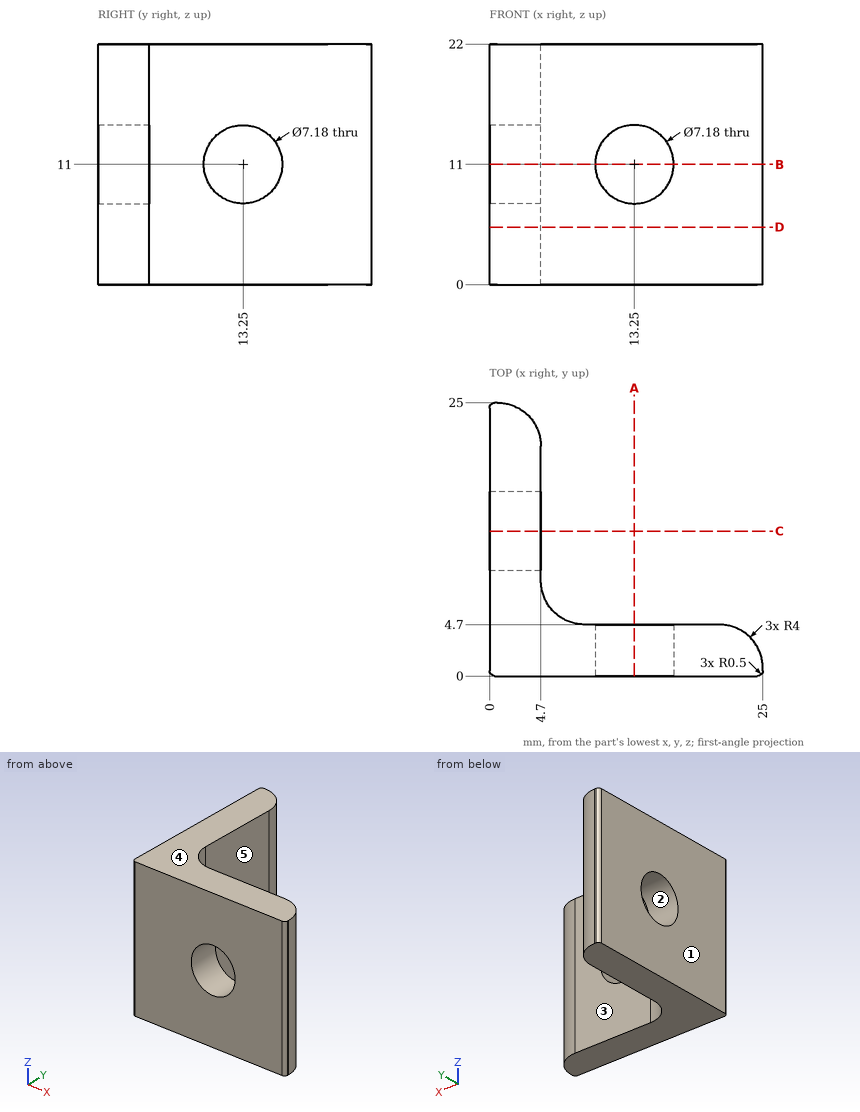
Source: three-view drawing plus pictorial views. Frame: mm from the lowest corner of the part. A direction names the side the tool comes from. Round coordinates to 2 decimals unless told otherwise and drop trailing zeros. Loops run counter-clockwise (first coordinate to the right, second up) from the corner with the lowest first, then second, coordinate; pieces in that order, holes last.
1. Contact query for flat-ended pins moving along their axis: pin 1 (5 mm diameter, centred on y = 16, z = 8, fed in from +X); pin 2 (4 mm diameter, centred on x = 8.5, z = 14.5, fed in from +Y); pin 3 (3.5 mm diameter, centred on x = 17, z = 11, fed in from +Y); pin 4 (5 mm diameter, centred on x = 19, y = 3, fed in from -Z). Output: stop coordinate, or through.
2. Mould query, pull axis Y, two halves, no side actions, for the marked faces 1, 2 and 3. Classes: released by +Y, released by -Y, zero draft, split by the parting line, or undercut.
3. Section query D-D on z = 5.25. Output: boundary loops of the cut face in (x, y), and give its area (3 significant figures).
4. Section query A-A on x = 13.25. Output: boundary loops of the cut face in (y, z).
5. Section query B-B on z = 11. Output: boundary loops of the cut face in (x, y).
6. Ray query, L1, parallel to Z at x = 3.05, y = 13.25; L2, parallel to X at y = 19.75, z = 6.75. Return the intervals inside material, ascending.
7. Access query for the marked faces 4 and 5. Directions: +Z, -Z, +X, -X, +Y, -Y. A direction counts if a zero-diameter tool reaches every point of the face in a straight line with its end or side. Return the directions, or none.
Answers below:
1. pin 1: stops at x = 4.7
1. pin 2: stops at y = 5.36
1. pin 3: stops at y = 4.7
1. pin 4: stops at z = 0
2. face 1: zero draft
2. face 2: undercut
2. face 3: released by +Y
3. outline: (0, 0.5) arc R0.5 ccw to (0.5, 0) - (24.5, 0) arc R0.5 ccw to (25, 0.5) - (25, 0.7) arc R4 ccw to (21, 4.7) - (8.7, 4.7) arc R4 cw to (4.7, 8.7) - (4.7, 21) arc R4 ccw to (0.7, 25) - (0.5, 25) arc R0.5 ccw to (0, 24.5) - close
3. area: 209 mm2
4. outline: (0, 0) - (4.7, 0) - (4.7, 7.41) - (0, 7.41) - close; (0, 14.59) - (4.7, 14.59) - (4.7, 22) - (0, 22) - close
5. outline: (0, 0.5) arc R0.5 ccw to (0.5, 0) - (9.66, 0) - (9.66, 4.7) - (8.7, 4.7) arc R4 cw to (4.7, 8.7) - (4.7, 9.66) - (0, 9.66) - close; (0, 16.84) - (4.7, 16.84) - (4.7, 21) arc R4 ccw to (0.7, 25) - (0.5, 25) arc R0.5 ccw to (0, 24.5) - close; (16.84, 0) - (24.5, 0) arc R0.5 ccw to (25, 0.5) - (25, 0.7) arc R4 ccw to (21, 4.7) - (16.84, 4.7) - close
6. L1: z = 0 to 7.41, 14.59 to 22
6. L2: x = 0 to 4.7
7. face 4: +Z, +X, -X, +Y, -Y
7. face 5: +Z, -Z, +X, +Y
